from build123d import *

# Parameters (mm, degrees)
SKETCH1_W           = 120
SKETCH1_H           = 80
BOSS_EXTRUDE1_DEPTH = 2
SKETCH1_3_W         = 124
SKETCH1_3_H         = 84
SKETCH1_3_W_2       = 120
SKETCH1_3_H_2       = 80
BOSS_EXTRUDE2_DEPTH = 52
SKETCH2_W           = 12
SKETCH2_H           = 16
CUT_EXTRUDE1_DEPTH  = 2
SKETCH3_R           = 2.5
CUT_EXTRUDE3_DEPTH  = 2
SKETCH5_R           = 5
SKETCH5_R_2         = 2.5
CUT_EXTRUDE6_DEPTH  = 2
FILLET1_R           = 5
FILLET2_R           = 5
FILLET3_R           = 5
FILLET4_R           = 5
BOSS_EXTRUDE3_DEPTH = 2


with BuildPart() as part:
    # Sketch1 → Boss-Extrude1 (new body)
    with BuildSketch(Plane(origin=(0, 0, 0), x_dir=(1, 0, 0), z_dir=(0, 1, 0))):
        Rectangle(SKETCH1_W, SKETCH1_H)
    extrude(amount=BOSS_EXTRUDE1_DEPTH)

    # Sketch1<3> → Boss-Extrude2 (add)
    with BuildSketch(Plane(origin=(0, 0, 0), x_dir=(1, 0, 0), z_dir=(0, 1, 0))):
        Rectangle(SKETCH1_3_W, SKETCH1_3_H)
        Rectangle(SKETCH1_3_W_2, SKETCH1_3_H_2, mode=Mode.SUBTRACT)
    extrude(amount=BOSS_EXTRUDE2_DEPTH)

    # Sketch2 → Cut-Extrude1 (cut)
    with BuildSketch(Plane.XY.offset(42)):
        with Locations((-39.5, 10)):
            Rectangle(SKETCH2_W, SKETCH2_H)
    extrude(amount=-CUT_EXTRUDE1_DEPTH, mode=Mode.SUBTRACT)

    # Sketch3 → Cut-Extrude3 (cut)
    with BuildSketch(Plane.XY.offset(42)):
        with Locations((29.5, 20)):
            Circle(SKETCH3_R)
    extrude(amount=-CUT_EXTRUDE3_DEPTH, mode=Mode.SUBTRACT)

    # Sketch5 → Cut-Extrude6 (cut)
    with BuildSketch(Plane(origin=(0, 0, -42), x_dir=(-1, 0, 0), z_dir=(0, 0, -1))):
        with Locations((-32, 20)):
            Circle(SKETCH5_R)
        with Locations((32, 20)):
            Circle(SKETCH5_R_2)
    extrude(amount=-CUT_EXTRUDE6_DEPTH, mode=Mode.SUBTRACT)

    # Fillet1
    fillet1_edges = [part.edges().sort_by_distance(p)[0] for p in [
        (62, 26, -42),
    ]]
    fillet(fillet1_edges, radius=FILLET1_R)

    # Fillet2
    fillet2_edges = [part.edges().sort_by_distance(p)[0] for p in [
        (62, 26, 42),
    ]]
    fillet(fillet2_edges, radius=FILLET2_R)

    # Fillet3
    fillet3_edges = [part.edges().sort_by_distance(p)[0] for p in [
        (-62, 26, -42),
    ]]
    fillet(fillet3_edges, radius=FILLET3_R)

    # Fillet4
    fillet4_edges = [part.edges().sort_by_distance(p)[0] for p in [
        (-62, 26, 42),
    ]]
    fillet(fillet4_edges, radius=FILLET4_R)

    # Sketch6 → Boss-Extrude3 (add)
    with BuildSketch(Plane(origin=(0, 52, 0), x_dir=(1, 0, 0), z_dir=(0, 1, 0))):
        Polygon((-50, 40), (-60, 30), (-60, 40), align=None)
        Polygon((-60, -30), (-60, -40), (-50, -40), align=None)
        Polygon((50, -40), (60, -30), (60, -40), align=None)
        Polygon((60, 30), (60, 40), (50, 40), align=None)
    extrude(amount=-BOSS_EXTRUDE3_DEPTH)


solid = part.part
Model file for the job. Use its own axes, mm. A direction names the side the tool comes from. Round coordinates to 2 decimals unless told otherwise and drop trailing zeros. Order: outer loops, then holes, each group sorted by start corner. A loop starts at its lowest first (then second) coordinate and runs counter-clockwise, first axis right, second up.
(1) Band-saw the part on A-A (y = 20). List the corners of the cut face in (x, z), then the cut area to 3 significant figures.
(2) Band-saw the part on D-D (z = 16). List the corners of the cut face in (x, y).
(3) 3-axis set-ups, long thin cutter, end or side, ignore diameter. For faces 1 (the face through (-57, 50, 37)), 2 (the face through (-1, 26, 42)), 3 (the face through (-55, 51, 35)), 4 (the face through (-31.67, 22.48, -41.01)), 5 (the face through (61, 26, 40)): which of +Z, -Z, +X, -X, +Y, -Y reach the whole face in a straight line?
(4) Band-saw the part on C-C (y = 31). List the corners of the cut face in (x, z), then the cut area to 3 significant figures.
(5) Drill centre lines: line 1 (X direction, y = 13, z = 14); line 2 (Y direction, x = 32, z = -41.3); line 3 (Z direction, x = -26.5, y = 9.5). Where is each one in solid material? Low to high.
(6) Pull direction X, two halves, no side cores. Call faces 6 (the face through (62, 26, 1)), 7 (the face through (29.17, 22.48, 41.01)), 8 (the face through (-1, 26, -42)): released by +X, released by -X, zero draft, split by the parting line, or undercut.
(7) Pin check, flat tips, straight feed: pin 1 (1 mm diameter, centred on x = -14.5, z = -12, fed in from +Y); pin 2 (4 mm diameter, centred on x = 29.5, y = 20, fed in from +Z); pin 3 (1.6 mm diameter, centred on y = 9, z = 41, fed in from -X); pin 4 (1 mm diameter, centred on y = 10, z = 41, fed in from +X). Stop position of each tip, or through.
(8) Band-saw the part on B-B (x = -32). List the corners of the cut face in (y, z), then the cut area to 3 significant figures.
Verdict:
1. outline: (-62, -37) arc R5 ccw to (-57, -42) - (-34.5, -42) - (-34.5, -40) - (-60, -40) - (-60, 40) - (27, 40) - (27, 42) - (-57, 42) arc R5 ccw to (-62, 37) - close; (-29.5, -42) - (27, -42) - (27, -40) - (-29.5, -40) - close; (32, 40) - (60, 40) - (60, -40) - (37, -40) - (37, -42) - (57, -42) arc R5 ccw to (62, -37) - (62, 37) arc R5 ccw to (57, 42) - (32, 42) - close
1. area: 755 mm2
2. outline: (-62, 0) - (62, 0) - (62, 52) - (60, 52) - (60, 2) - (-60, 2) - (-60, 52) - (-62, 52) - close
3. face 1: none
3. face 2: +Z, +X, -X, +Y, -Y
3. face 3: +Y
3. face 4: -Z
3. face 5: +Z, +X, +Y, -Y
4. outline: (-62, -37) arc R5 ccw to (-57, -42) - (57, -42) arc R5 ccw to (62, -37) - (62, 37) arc R5 ccw to (57, 42) - (-57, 42) arc R5 ccw to (-62, 37) - close; hole (-60, -40) - (60, -40) - (60, 40) - (-60, 40) - close
4. area: 795 mm2
5. line 1: x = -62 to -60, 60 to 62
5. line 2: y = 0 to 15, 25 to 52
5. line 3: z = -42 to -40, 40 to 42
6. face 6: released by +X
6. face 7: undercut
6. face 8: zero draft
7. pin 1: stops at y = 2
7. pin 2: passes through
7. pin 3: stops at x = -60.84
7. pin 4: stops at x = 60.57
8. outline: (0, -42) - (17.5, -42) - (17.5, -40) - (2, -40) - (2, 40) - (52, 40) - (52, 42) - (0, 42) - close; (22.5, -42) - (52, -42) - (52, -40) - (22.5, -40) - close
8. area: 358 mm2
